```python
from build123d import *

# Parameters (mm, degrees)
F0_W     = 120
F0_H     = 80
F0_R     = 25
F1_DEPTH = 50
F3_DEPTH = 25


with BuildPart() as f1:
    # F0 (on Front) → F1 (new body)
    with BuildSketch(Plane.XZ):
        Rectangle(F0_W, F0_H)
        Circle(F0_R, mode=Mode.SUBTRACT)
    extrude(amount=F1_DEPTH)

    # F2 (on face) → F3 (cut)
    with BuildSketch(Plane.XZ.offset(50)):
        Polygon((60, -40), (60, 40), (-20, 40), (30, -40), align=None)
    extrude(amount=-F3_DEPTH, mode=Mode.SUBTRACT)


solid = f1.part
```
Check sheet for the modelled part. Datum: model origin and axes. Units: mm. A direction names the side the tool comes from. Coordinates: 2 decimals unless noted, no trailing zeros. Order: outer loops, then holes, each group sorted by start corner. A loop starts at its lowest first (then second) coordinate and runs counter-clockwise, first axis right, second up. Notation, with made-up numbers: M 32,-16.75 L 37,-16.75 A32 cw 37,21.25 Z; hole C 16.25,-14.5 d7. An arc over 180 degrees is marked long. Write each question's results on one line, items separated by ' | '. Start each with the question number.
1. Material ranges on probe 1 along X at (y, z) = (-9, 0); probe 2 along Z at (x, y) = (0, -24); probe 3 along Z at (x, y) = (0, -32), recorded low to high.
2. Access from +Z, -Z, +X, -X, +Y, -Y to the whole of each face (thin tool, end or side, straight path). Record for faces 4 (the face through (-1, -25, -40)), 5 (the face through (-15, -38, 32)).
3. Cross-section at C-C on y = -10. Record the cut outline in (x, z), and give its area (3 significant figures).
4. Go/stop test with flat-tipped pins: P1, Ø1, axis at y = -28, z = -21.5, coming from the +X side; P2, Ø3, axis at y = -37.5, z = 19.5, coming from the +X side. Record where each tip stops, or that it passes through.
5. Cross-section at A-A on z = 20. Record the cut outline in (x, y), and give its area (4 significant figures).
6. Cross-section at B-B on x = 0. Record the cut outline in (y, z), and give its area (4 significant figures).
7. Mould release check, pull along Z, two halves, no side actions. Record for faces 1 (the face through (-14, -19, 40)), 2 (the face through (60, -12, -1)), 3 (the face through (-20, -19, -15)): +Z half, -Z half, draft (parallel to the pull), parting line (faces both ways), or undercut.
8. Cross-section at D-D on z = 32. Record the cut outline in (x, y).
Checks:
1) probe 1: x = -60 to -25, 25 to 60 | probe 2: z = -40 to -25, 25 to 40 | probe 3: z = -40 to -25
2) face 4: -Z, +X, -X, +Y, -Y | face 5: +Z, +X, -Y
3) outline: M -60,-40 L 60,-40 L 60,40 L -60,40 Z; hole C 0,0 d50 | area: 7,640 mm²
4) P1: stops at x = 18.75 | P2: stops at x = -13.56
5) outline: M -60,-50 L -15,-50 L -15,0 L -60,0 Z; M 15,-25 L 60,-25 L 60,0 L 15,0 Z | area: 3,375 mm²
6) outline: M -50,-40 L 0,-40 L 0,-25 L -50,-25 Z; M -25,25 L 0,25 L 0,40 L -25,40 Z | area: 1,125 mm²
7) face 1: +Z half | face 2: draft | face 3: undercut
8) outline: M -60,-50 L -15,-50 L -15,-25 L 60,-25 L 60,0 L -60,0 Z
